CAD build for the part. Positions are in the model's coordinates, mm. Give positions to 0.01 mm unless a question says otherwise; leave off trailing zeros. Loops run counter-clockwise (first coordinate to the right, second up) from the corner with the lowest first, then second, coordinate; pieces in that order, holes last.
```python
from build123d import *

# Parameters (mm, degrees)
SKETCH1_W           = 17.78
SKETCH1_H           = 10.16
BOSS_EXTRUDE1_DEPTH = 1.5875
SKETCH2_W           = 3.1
SKETCH2_H           = 2.1
BOSS_EXTRUDE2_DEPTH = 0.8
CUT_EXTRUDE1_REACH  = 12.361
SKETCH3_R           = 0.635


with BuildPart() as part:
    # Sketch1 → Boss-Extrude1 (new body)
    with BuildSketch(Plane(origin=(0, 0, 0), x_dir=(1, 0, 0), z_dir=(0, 1, 0))):
        Rectangle(SKETCH1_W, SKETCH1_H)
    extrude(amount=-BOSS_EXTRUDE1_DEPTH)

    # Sketch2 → Boss-Extrude2 (add)
    with BuildSketch(Plane(origin=(0, 0, 0), x_dir=(1, 0, 0), z_dir=(0, 1, 0))):
        Rectangle(SKETCH2_W, SKETCH2_H)
    extrude(amount=BOSS_EXTRUDE2_DEPTH)

    # Sketch3 → Cut-Extrude1 (cut, up to next)
    with BuildSketch(Plane(origin=(0, 0, 0), x_dir=(1, 0, 0), z_dir=(0, 1, 0)), mode=Mode.PRIVATE) as cut_extrude1_sk1:
        with Locations(Location((-7.62, 3.81, 0), (0, 0, 270))):
            Circle(SKETCH3_R)
    cut_extrude1_tool1 = extrude(cut_extrude1_sk1.sketch, amount=-CUT_EXTRUDE1_REACH, mode=Mode.PRIVATE) & part.part
    # Sketch3 → Cut-Extrude1 (cut, up to next)
    with BuildSketch(Plane(origin=(0, 0, 0), x_dir=(1, 0, 0), z_dir=(0, 1, 0)), mode=Mode.PRIVATE) as cut_extrude1_sk2:
        with Locations(Location((-7.62, -3.81, 0), (0, 0, 270))):
            Circle(SKETCH3_R)
    cut_extrude1_tool2 = extrude(cut_extrude1_sk2.sketch, amount=-CUT_EXTRUDE1_REACH, mode=Mode.PRIVATE) & part.part
    # Sketch3 → Cut-Extrude1 (cut, up to next)
    with BuildSketch(Plane(origin=(0, 0, 0), x_dir=(1, 0, 0), z_dir=(0, 1, 0)), mode=Mode.PRIVATE) as cut_extrude1_sk3:
        with Locations(Location((-5.08, 3.81, 0), (0, 0, 270))):
            Circle(SKETCH3_R)
    cut_extrude1_tool3 = extrude(cut_extrude1_sk3.sketch, amount=-CUT_EXTRUDE1_REACH, mode=Mode.PRIVATE) & part.part
    # Sketch3 → Cut-Extrude1 (cut, up to next)
    with BuildSketch(Plane(origin=(0, 0, 0), x_dir=(1, 0, 0), z_dir=(0, 1, 0)), mode=Mode.PRIVATE) as cut_extrude1_sk4:
        with Locations(Location((-5.08, -3.81, 0), (0, 0, 270))):
            Circle(SKETCH3_R)
    cut_extrude1_tool4 = extrude(cut_extrude1_sk4.sketch, amount=-CUT_EXTRUDE1_REACH, mode=Mode.PRIVATE) & part.part
    # Sketch3 → Cut-Extrude1 (cut, up to next)
    with BuildSketch(Plane(origin=(0, 0, 0), x_dir=(1, 0, 0), z_dir=(0, 1, 0)), mode=Mode.PRIVATE) as cut_extrude1_sk5:
        with Locations(Location((-2.54, 3.81, 0), (0, 0, 270))):
            Circle(SKETCH3_R)
    cut_extrude1_tool5 = extrude(cut_extrude1_sk5.sketch, amount=-CUT_EXTRUDE1_REACH, mode=Mode.PRIVATE) & part.part
    # Sketch3 → Cut-Extrude1 (cut, up to next)
    with BuildSketch(Plane(origin=(0, 0, 0), x_dir=(1, 0, 0), z_dir=(0, 1, 0)), mode=Mode.PRIVATE) as cut_extrude1_sk6:
        with Locations(Location((-2.54, -3.81, 0), (0, 0, 270))):
            Circle(SKETCH3_R)
    cut_extrude1_tool6 = extrude(cut_extrude1_sk6.sketch, amount=-CUT_EXTRUDE1_REACH, mode=Mode.PRIVATE) & part.part
    # Sketch3 → Cut-Extrude1 (cut, up to next)
    with BuildSketch(Plane(origin=(0, 0, 0), x_dir=(1, 0, 0), z_dir=(0, 1, 0)), mode=Mode.PRIVATE) as cut_extrude1_sk7:
        with Locations(Location((0, 3.81, 0), (0, 0, 270))):
            Circle(SKETCH3_R)
    cut_extrude1_tool7 = extrude(cut_extrude1_sk7.sketch, amount=-CUT_EXTRUDE1_REACH, mode=Mode.PRIVATE) & part.part
    # Sketch3 → Cut-Extrude1 (cut, up to next)
    with BuildSketch(Plane(origin=(0, 0, 0), x_dir=(1, 0, 0), z_dir=(0, 1, 0)), mode=Mode.PRIVATE) as cut_extrude1_sk8:
        with Locations(Location((0, -3.81, 0), (0, 0, 270))):
            Circle(SKETCH3_R)
    cut_extrude1_tool8 = extrude(cut_extrude1_sk8.sketch, amount=-CUT_EXTRUDE1_REACH, mode=Mode.PRIVATE) & part.part
    # Sketch3 → Cut-Extrude1 (cut, up to next)
    with BuildSketch(Plane(origin=(0, 0, 0), x_dir=(1, 0, 0), z_dir=(0, 1, 0)), mode=Mode.PRIVATE) as cut_extrude1_sk9:
        with Locations(Location((2.54, 3.81, 0), (0, 0, 270))):
            Circle(SKETCH3_R)
    cut_extrude1_tool9 = extrude(cut_extrude1_sk9.sketch, amount=-CUT_EXTRUDE1_REACH, mode=Mode.PRIVATE) & part.part
    # Sketch3 → Cut-Extrude1 (cut, up to next)
    with BuildSketch(Plane(origin=(0, 0, 0), x_dir=(1, 0, 0), z_dir=(0, 1, 0)), mode=Mode.PRIVATE) as cut_extrude1_sk10:
        with Locations(Location((2.54, -3.81, 0), (0, 0, 270))):
            Circle(SKETCH3_R)
    cut_extrude1_tool10 = extrude(cut_extrude1_sk10.sketch, amount=-CUT_EXTRUDE1_REACH, mode=Mode.PRIVATE) & part.part
    # Sketch3 → Cut-Extrude1 (cut, up to next)
    with BuildSketch(Plane(origin=(0, 0, 0), x_dir=(1, 0, 0), z_dir=(0, 1, 0)), mode=Mode.PRIVATE) as cut_extrude1_sk11:
        with Locations(Location((5.08, 3.81, 0), (0, 0, 270))):
            Circle(SKETCH3_R)
    cut_extrude1_tool11 = extrude(cut_extrude1_sk11.sketch, amount=-CUT_EXTRUDE1_REACH, mode=Mode.PRIVATE) & part.part
    # Sketch3 → Cut-Extrude1 (cut, up to next)
    with BuildSketch(Plane(origin=(0, 0, 0), x_dir=(1, 0, 0), z_dir=(0, 1, 0)), mode=Mode.PRIVATE) as cut_extrude1_sk12:
        with Locations(Location((5.08, -3.81, 0), (0, 0, 270))):
            Circle(SKETCH3_R)
    cut_extrude1_tool12 = extrude(cut_extrude1_sk12.sketch, amount=-CUT_EXTRUDE1_REACH, mode=Mode.PRIVATE) & part.part
    # Sketch3 → Cut-Extrude1 (cut, up to next)
    with BuildSketch(Plane(origin=(0, 0, 0), x_dir=(1, 0, 0), z_dir=(0, 1, 0)), mode=Mode.PRIVATE) as cut_extrude1_sk13:
        with Locations(Location((7.62, 3.81, 0), (0, 0, 270))):
            Circle(SKETCH3_R)
    cut_extrude1_tool13 = extrude(cut_extrude1_sk13.sketch, amount=-CUT_EXTRUDE1_REACH, mode=Mode.PRIVATE) & part.part
    # Sketch3 → Cut-Extrude1 (cut, up to next)
    with BuildSketch(Plane(origin=(0, 0, 0), x_dir=(1, 0, 0), z_dir=(0, 1, 0)), mode=Mode.PRIVATE) as cut_extrude1_sk14:
        with Locations(Location((7.62, -3.81, 0), (0, 0, 270))):
            Circle(SKETCH3_R)
    cut_extrude1_tool14 = extrude(cut_extrude1_sk14.sketch, amount=-CUT_EXTRUDE1_REACH, mode=Mode.PRIVATE) & part.part
    add(cut_extrude1_tool1.solids().sort_by_distance((-7.62, 0, -3.81))[0], mode=Mode.SUBTRACT)
    add(cut_extrude1_tool2.solids().sort_by_distance((-7.62, 0, 3.81))[0], mode=Mode.SUBTRACT)
    add(cut_extrude1_tool3.solids().sort_by_distance((-5.08, 0, -3.81))[0], mode=Mode.SUBTRACT)
    add(cut_extrude1_tool4.solids().sort_by_distance((-5.08, 0, 3.81))[0], mode=Mode.SUBTRACT)
    add(cut_extrude1_tool5.solids().sort_by_distance((-2.54, 0, -3.81))[0], mode=Mode.SUBTRACT)
    add(cut_extrude1_tool6.solids().sort_by_distance((-2.54, 0, 3.81))[0], mode=Mode.SUBTRACT)
    add(cut_extrude1_tool7.solids().sort_by_distance((0, 0, -3.81))[0], mode=Mode.SUBTRACT)
    add(cut_extrude1_tool8.solids().sort_by_distance((0, 0, 3.81))[0], mode=Mode.SUBTRACT)
    add(cut_extrude1_tool9.solids().sort_by_distance((2.54, 0, -3.81))[0], mode=Mode.SUBTRACT)
    add(cut_extrude1_tool10.solids().sort_by_distance((2.54, 0, 3.81))[0], mode=Mode.SUBTRACT)
    add(cut_extrude1_tool11.solids().sort_by_distance((5.08, 0, -3.81))[0], mode=Mode.SUBTRACT)
    add(cut_extrude1_tool12.solids().sort_by_distance((5.08, 0, 3.81))[0], mode=Mode.SUBTRACT)
    add(cut_extrude1_tool13.solids().sort_by_distance((7.62, 0, -3.81))[0], mode=Mode.SUBTRACT)
    add(cut_extrude1_tool14.solids().sort_by_distance((7.62, 0, 3.81))[0], mode=Mode.SUBTRACT)


solid = part.part
```
1. Saw through at A-A, the plane z = -3.81. Count the separate pieces of the cut face and the enclosed holes in it, and give its area (3 significant figures).
Responses:
separate pieces: 8
enclosed holes: 0
area: 14.1 mm2
2. Saw through at D-D, the plane x = -2.54. List the corners of the cut face in (y, z) (1 decimal), and give its area (3 significant figures).
Responses:
outline: (-1.6, -5.1) - (0, -5.1) - (0, -4.4) - (-1.6, -4.4) - close; (-1.6, -3.2) - (0, -3.2) - (0, 3.2) - (-1.6, 3.2) - close; (-1.6, 4.4) - (0, 4.4) - (0, 5.1) - (-1.6, 5.1) - close
area: 12.1 mm2
3. Pull direction X, two halves, no side cores. Call faces 1 (the face through (0, -1.588, 0)), 2 (the face through (0.191, -0.783, -3.204)), 3 (the face through (1.977, -0.783, -3.517)), 4 (the face through (-8.89, -1, 0)): released by +X, released by -X, zero draft, split by the parting line, or undercut.
Responses:
face 1: zero draft
face 2: undercut
face 3: undercut
face 4: released by -X
4. Drop a flat-ended pin along its axis: pin 1 (1.7 mm diameter, centred on x = 5.08, z = -3.81, fed in from +Y). Give the stop position or say it passes through.
Responses:
pin 1: stops at y = 0
5. Probe line 1 along Z through (x, y) = (-5, -0.7); line 2 along Z through (x, y) = (-3, -0.1); line 3 along Y through (x, z) = (-4, 1.25). List the from-to ranges inside material, lowest first.
Responses:
line 1: z = -5.08 to -4.44, -3.18 to 3.18, 4.44 to 5.08
line 2: z = -5.08 to -4.25, -3.37 to 3.37, 4.25 to 5.08
line 3: y = -1.59 to 0
